```python
from build123d import *

# Parameters (mm, degrees)
F2_DEPTH  = 13.5
F2_TAPER  = -55
F4_DEPTH  = 19
F4_TAPER  = -33
F6_DEPTH  = 24
F6_TAPER  = -11.5
F8_DEPTH  = 24
F8_TAPER  = 11.5
F10_DEPTH = 19
F10_TAPER = 33
F12_DEPTH = 13.5
F12_TAPER = 55
F17_COUNT = 12
F17_ANGLE = 330
F19_W     = 150.1999571919
F19_H     = 155.7629220188
F20_DEPTH = 104.0525976479
F21_R     = 31.5
F22_DEPTH = 25
F23_R     = 31.5
F24_DEPTH = 5


with BuildPart() as f2:
    # F1 (on Top) → F2 (new body)
    with BuildSketch(Plane.XY):
        Polygon((18.667295593, -18.667295593), (25.5, -6.832704407), (25.5, 6.832704407), (18.667295593, 18.667295593), (6.832704407, 25.5), (-6.832704407, 25.5), (-18.667295593, 18.667295593), (-25.5, 6.832704407), (-25.5, -6.832704407), (-18.667295593, -18.667295593), (-6.832704407, -25.5), (6.832704407, -25.5), align=None)
    extrude(amount=F2_DEPTH, taper=F2_TAPER)

    # F3 (on face) → F4 (join)
    with BuildSketch(Plane.XY.offset(13.5)):
        Polygon((11.9987643256, -44.779998091), (32.7812337655, -32.7812337655), (44.779998091, -11.9987643256), (44.779998091, 11.9987643256), (32.7812337655, 32.7812337655), (11.9987643256, 44.779998091), (-11.9987643256, 44.779998091), (-32.7812337655, 32.7812337655), (-44.779998091, 11.9987643256), (-44.779998091, -11.9987643256), (-32.7812337655, -32.7812337655), (-11.9987643256, -44.779998091), align=None)
    extrude(amount=F4_DEPTH, taper=F4_TAPER)

    # F5 (on face) → F6 (join)
    with BuildSketch(Plane.XY.offset(32.5)):
        Polygon((15.3049208885, -57.1187423618), (41.8138214733, -41.8138214733), (57.1187423618, -15.3049208885), (57.1187423618, 15.3049208885), (41.8138214733, 41.8138214733), (15.3049208885, 57.1187423618), (-15.3049208885, 57.1187423618), (-41.8138214733, 41.8138214733), (-57.1187423618, 15.3049208885), (-57.1187423618, -15.3049208885), (-41.8138214733, -41.8138214733), (-15.3049208885, -57.1187423618), align=None)
    extrude(amount=F6_DEPTH, taper=F6_TAPER)

    # F7 (on face) → F8 (join)
    with BuildSketch(Plane.XY.offset(56.5)):
        Polygon((-16.6132779924, -62.0015975479), (16.6132779924, -62.0015975479), (45.3883195555, -45.3883195555), (62.0015975479, -16.6132779924), (62.0015975479, 16.6132779924), (45.3883195555, 45.3883195555), (16.6132779924, 62.0015975479), (-16.6132779924, 62.0015975479), (-45.3883195555, 45.3883195555), (-62.0015975479, 16.6132779924), (-62.0015975479, -16.6132779924), (-45.3883195555, -45.3883195555), align=None)
    extrude(amount=F8_DEPTH, taper=F8_TAPER)

    # F9 (on face) → F10 (join)
    with BuildSketch(Plane.XY.offset(80.5)):
        Polygon((15.3049208885, -57.1187423618), (41.8138214733, -41.8138214733), (57.1187423618, -15.3049208885), (57.1187423618, 15.3049208885), (41.8138214733, 41.8138214733), (15.3049208885, 57.1187423618), (-15.3049208885, 57.1187423618), (-41.8138214733, 41.8138214733), (-57.1187423618, 15.3049208885), (-57.1187423618, -15.3049208885), (-41.8138214733, -41.8138214733), (-15.3049208885, -57.1187423618), align=None)
    extrude(amount=F10_DEPTH, taper=F10_TAPER)

    # F11 (on face) → F12 (join)
    with BuildSketch(Plane.XY.offset(99.5)):
        Polygon((-32.7812337655, -32.7812337655), (-11.9987643256, -44.779998091), (11.9987643256, -44.779998091), (32.7812337655, -32.7812337655), (44.779998091, -11.9987643256), (44.779998091, 11.9987643256), (32.7812337655, 32.7812337655), (11.9987643256, 44.779998091), (-11.9987643256, 44.779998091), (-32.7812337655, 32.7812337655), (-44.779998091, 11.9987643256), (-44.779998091, -11.9987643256), align=None)
    extrude(amount=F12_DEPTH, taper=F12_TAPER)


with BuildPart() as f16:
    # F15 (on 3pt) → F16 (new body, up to the next surface of F2)
    with BuildSketch(Plane(origin=(12.3175443523, -21.3346126427, 113.1882453996), x_dir=(0.9943304543, 0.0196958746, -0.1044941158), z_dir=(-0.1063341323, 0.1841761198, -0.9771244594))):
        Polygon((6.3859567143, -2.5862935324), (-5.5161138048, 4.1281770657), (-12.3877774228, -21.9585741432), align=None)
    extrude(until=Until.NEXT, target=f2.part)


with BuildPart() as f17_1:
    # F17: instance of F16
    add(f16.part.rotate(Axis((0, 0, 87.5846954226), (0, 0, 1)), 1 * F17_ANGLE / (F17_COUNT - 1)))


with BuildPart() as f17_2:
    # F17: instance of F16
    add(f16.part.rotate(Axis((0, 0, 87.5846954226), (0, 0, 1)), 2 * F17_ANGLE / (F17_COUNT - 1)))


with BuildPart() as f17_3:
    # F17: instance of F16
    add(f16.part.rotate(Axis((0, 0, 87.5846954226), (0, 0, 1)), 3 * F17_ANGLE / (F17_COUNT - 1)))


with BuildPart() as f17_4:
    # F17: instance of F16
    add(f16.part.rotate(Axis((0, 0, 87.5846954226), (0, 0, 1)), 4 * F17_ANGLE / (F17_COUNT - 1)))


with BuildPart() as f17_5:
    # F17: instance of F16
    add(f16.part.rotate(Axis((0, 0, 87.5846954226), (0, 0, 1)), 5 * F17_ANGLE / (F17_COUNT - 1)))


with BuildPart() as f17_6:
    # F17: instance of F16
    add(f16.part.rotate(Axis((0, 0, 87.5846954226), (0, 0, 1)), 6 * F17_ANGLE / (F17_COUNT - 1)))


with BuildPart() as f17_7:
    # F17: instance of F16
    add(f16.part.rotate(Axis((0, 0, 87.5846954226), (0, 0, 1)), 7 * F17_ANGLE / (F17_COUNT - 1)))


with BuildPart() as f17_8:
    # F17: instance of F16
    add(f16.part.rotate(Axis((0, 0, 87.5846954226), (0, 0, 1)), 8 * F17_ANGLE / (F17_COUNT - 1)))


with BuildPart() as f17_9:
    # F17: instance of F16
    add(f16.part.rotate(Axis((0, 0, 87.5846954226), (0, 0, 1)), 9 * F17_ANGLE / (F17_COUNT - 1)))


with BuildPart() as f17_10:
    # F17: instance of F16
    add(f16.part.rotate(Axis((0, 0, 87.5846954226), (0, 0, 1)), 10 * F17_ANGLE / (F17_COUNT - 1)))


with BuildPart() as f17_11:
    # F17: instance of F16
    add(f16.part.rotate(Axis((0, 0, 87.5846954226), (0, 0, 1)), 11 * F17_ANGLE / (F17_COUNT - 1)))


with BuildPart() as f20_tool:
    # F19 (on offset) → F20 (new body, through all)
    with BuildSketch(Plane.XZ.offset(42.05)):
        with Locations((3.019284457, 52.1549973637)):
            Rectangle(F19_W, F19_H)
    extrude(amount=-F20_DEPTH)


with BuildPart() as f2_1:
    add(f2.part)

    # F20: cut by f20_tool
    add(f20_tool.part, mode=Mode.SUBTRACT)

    # F21 (on face) → F22 (cut)
    with BuildSketch(Plane(origin=(0, -42.05, 0), x_dir=(-1, 0, 0), z_dir=(0, 1, 0))):
        with Locations((0, 56.5)):
            Circle(F21_R)
    extrude(amount=-F22_DEPTH, mode=Mode.SUBTRACT)

    # F23 (on face) → F24 (cut)
    with BuildSketch(Plane(origin=(0, -42.05, 0), x_dir=(-1, 0, 0), z_dir=(0, 1, 0))):
        Polygon((13, 92), (-13, 92), (-35.5, 69.5), (-35.5, 43.5), (-13, 21), (13, 21), (35.5, 43.5), (35.5, 56.5), (35.5, 69.5), align=None)
        with Locations((0, 56.5)):
            Circle(F23_R, mode=Mode.SUBTRACT)
    extrude(amount=-F24_DEPTH, mode=Mode.SUBTRACT)


with BuildPart() as f16_1:
    add(f16.part)

    # F20: cut by f20_tool
    add(f20_tool.part, mode=Mode.SUBTRACT)


with BuildPart() as f17_1_1:
    add(f17_1.part)

    # F20: cut by f20_tool
    add(f20_tool.part, mode=Mode.SUBTRACT)


with BuildPart() as f17_2_1:
    add(f17_2.part)

    # F20: cut by f20_tool
    add(f20_tool.part, mode=Mode.SUBTRACT)


with BuildPart() as f17_3_1:
    add(f17_3.part)

    # F20: cut by f20_tool
    add(f20_tool.part, mode=Mode.SUBTRACT)


with BuildPart() as f17_4_1:
    add(f17_4.part)

    # F20: cut by f20_tool
    add(f20_tool.part, mode=Mode.SUBTRACT)


with BuildPart() as f17_5_1:
    add(f17_5.part)

    # F20: cut by f20_tool
    add(f20_tool.part, mode=Mode.SUBTRACT)


with BuildPart() as f17_6_1:
    add(f17_6.part)

    # F20: cut by f20_tool
    add(f20_tool.part, mode=Mode.SUBTRACT)


with BuildPart() as f17_7_1:
    add(f17_7.part)

    # F20: cut by f20_tool
    add(f20_tool.part, mode=Mode.SUBTRACT)


with BuildPart() as f17_8_1:
    add(f17_8.part)

    # F20: cut by f20_tool
    add(f20_tool.part, mode=Mode.SUBTRACT)


with BuildPart() as f17_9_1:
    add(f17_9.part)

    # F20: cut by f20_tool
    add(f20_tool.part, mode=Mode.SUBTRACT)


with BuildPart() as f17_10_1:
    add(f17_10.part)

    # F20: cut by f20_tool
    add(f20_tool.part, mode=Mode.SUBTRACT)


with BuildPart() as f17_11_1:
    add(f17_11.part)

    # F20: cut by f20_tool
    add(f20_tool.part, mode=Mode.SUBTRACT)


solid = f2_1.part
```
The listing builds one solid part. Answer for the finished solid, in the listing's coordinates (mm). A direction names the side the tool comes from. Coordinates: 2 decimals unless noted, no trailing zeros. Loops run counter-clockwise (first coordinate to the right, second up) from the corner with the lowest first, then second, coordinate; pieces in that order, holes last. Notation, with made-up numbers: M 57,-22.75 L 85,-22.75 A29 ccw 85,7.25 Z; hole C -11,60.5 d7. An arc over 180 degrees is marked long. Answer as a JSON object with one key per item and string values. Group by question number.
Item 1: Section A-A (z = 71) is taken. Write down the section's boundary in (x, y), and give its area (3 significant figures).
Item 2: Section C-C (z = 83) is taken. Write down the section's boundary in (x, y), and give its area (3 significant figures).
Item 3: Section B-B (y = -52) is taken. Give the number of separate pieces and of enclosed holes in the cut face, and give its area (3 significant figures).
Item 4: Which of the six approach directions +Z, -Z, +X, -X, +Y, -Y give full straight-line access (tool end or side, diameter ignored) to faces 1 (the face through (-35.26, -48.457, 68.332)), 2 (the face through (35.5, -45, 57))?
Item 5: Determine the mould class of faces 3 (the face through (0.168, -43.434, 100.442)), 4 (the face through (0, -45, 92)), 5 (the face through (-23.28, -47.07, 87.76)), 6 (the face through (44.64, -43.2, 65.06)) for opening direction X: +X half, -X half, draft (parallel to the pull), parting line (faces both ways), or undercut.
Item 6: Consider L1, parallel to X at y = -50.5, z = 56.5; L2, parallel to Z at x = -26, y = -45.5; L3, parallel to X at y = -45, z = 84. Determine where each line is inside the solid, lowest interval first.
Item 7: Each of these flat-tipped pins is pushed along its axis until it touches: P1, Ø1.5, axis at x = 2, y = -53, coming from the +Z side; P2, Ø8, axis at x = 28.5, z = 67, coming from the -Y side; P3, Ø5.5, axis at y = -43.5, z = 60, coming from the +X side. Where does it stop, or does it pass through?
Solved:
{
 "1": {"outline": "M -43.91,-42.05 L -43.23,-43.23 L -27.96,-52.04 L -27.96,-47.05 L -34,-47.05 L -34,-42.05 Z; M 27.96,-52.04 L 43.23,-43.23 L 43.91,-42.05 L 34,-42.05 L 34,-47.05 L 27.96,-47.05 Z", "area": "111 mm2"},
 "2": {"outline": "M -38.16,-42.05 L -17.03,-54.25 L -17.03,-47.05 L -22,-47.05 L -22,-42.05 Z; M 17.03,-54.25 L 38.16,-42.05 L 22,-42.05 L 22,-47.05 L 17.03,-47.05 Z", "area": "208 mm2"},
 "3": {"separate pieces": "4", "enclosed holes": "0", "area": "273 mm2"},
 "4": {"face 1": "+Z, -X, -Y", "face 2": "+Y"},
 "5": {"face 3": "draft", "face 4": "undercut", "face 5": "-X half", "face 6": "+X half"},
 "6": {"L1": "x = -36.53 to -31.5, 31.5 to 36.53", "L2": "z = 25.24 to 34, 79 to 87.76", "L3": "x = -31.75 to -21, 21 to 31.75"},
 "7": {"P1": "stops at z = 88", "P2": "stops at y = -52.2", "P3": "stops at x = 47.04"}
}
